Geometry: final body of the model. Coordinates: model frame, mm. Face numbers are marked on the shaded views. A direction names the side the tool comes from. Round coordinates to 2 decimals unless told otherwise and drop trailing zeros. Order: outer loops, then holes, each group sorted by start corner. A loop starts at its lowest first (then second) coordinate and runs counter-clockwise, first axis right, second up. Notation, with made-up numbers: M 18,-38.75 L 42,-38.75 A34 cw 42,-3.75 Z; hole C -34.75,89 d1. An arc over 180 degrees is marked long. Return JSON: item names as keys, results as strings. Group by question number.
Q1. Contact query for flat-ended pins moving along their axis: pin 1 (1.8 mm diameter, centred on x = -3.5, y = -0.5, fed in from -Z); pin 2 (4 mm diameter, centred on x = 1.5, z = -2.5, fed in from +Y); pin 3 (1.5 mm diameter, centred on x = 4, z = 1, fed in from -Y); pin 4 (4 mm diameter, centred on x = 4.5, y = 1.5, fed in from -Z). Output: stop coordinate, or through.
Q2. Access query for the marked faces 4, 5 and 6. Directions: +Z, -Z, +X, -X, +Y, -Y. A direction counts if a zero-diameter tool reaches every point of the face in a straight line with its end or side. Return the directions, or none.
Q3. Cut plane A-A on x = 9.25. Output: boundary loops of the cut face in (y, z), and give its area (3 significant figures).
Q4. Ray query, probe 1 along Z at (x, y) = (-3.5, 0); probe 2 along X at (y, z) = (-2.25, 1.25); probe 3 along X at (y, z) = (2, 0). Return the intervals inside material, ascending.
Q5. Mould query, pull axis Y, two halves, no side actions, for the marked faces 1, 2 and 3. Classes: released by +Y, released by -Y, zero draft, split by the parting line, or undercut.
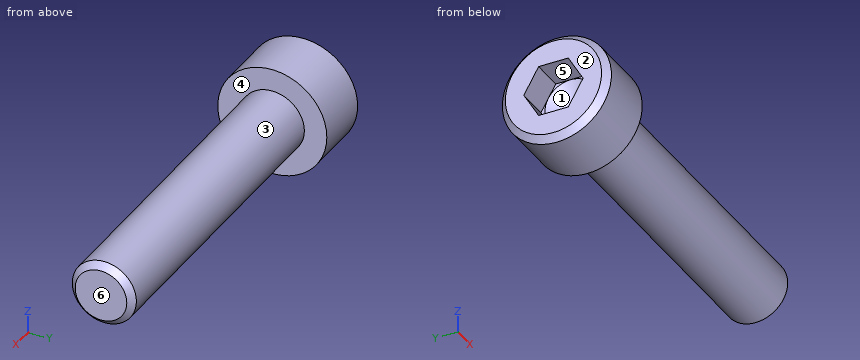
Autodesk Inventor part; units mm, degrees
ref_plane "bolt_XY" through (25, 0, 0) normal (1, 0, 0) x (0, 0, -1)
ref_plane "bolt_YZ" through (25, 0, 0) normal (0, 0, -1) x (0, 1, 0)
ref_plane "bolt_ZX" through (25, 0, 0) normal (0, 1, 0) x (1, 0, 0)
sketch "Sketch_1" plane through (0, 0, 0) normal (0, 0, 1) x (1, 0, 0)
  line L0 (25, 0) -> (-5, 0)
  line L1 (-5, 0) -> (-5, 3.75)
  line L2 (-5, 3.75) -> (-4.5, 4.25)
  line L3 (-4.5, 4.25) -> (0, 4.25)
  line L4 (0, 4.25) -> (0, 2.5)
  line L5 (0, 2.5) -> (24.5095, 2.5)
  line L6 (24.5095, 2.5) -> (25, 2.0095)
  line L7 (25, 2.0095) -> (25, 0)
  line L8 (25, 0) -> (-5, 0)
revolve "Revolution1" add sketch "Sketch_1" angle 360 about axis through (25, 0, 0) along (1, 0, 0)
thread "Thread1"
sketch "Sketch2" plane through (-5, 0, 0) normal (-1, 0, 0) x (0, 0, 1)
  point P0 (0, 0)
hole "Hole1" at (-5, 0, 0) direction (1, 0, 0) diameter 4 depth 2.5 tip angle 120
sketch "Sketch_3" plane through (-5, 0, 0) normal (1, 0, 0) x (0, 0, -1)
  line L0 (-2, -1.1547) -> (0, -2.3094)
  line L1 (0, -2.3094) -> (2, -1.1547)
  line L2 (2, -1.1547) -> (2, 1.1547)
  line L3 (2, 1.1547) -> (0, 2.3094)
  line L4 (0, 2.3094) -> (-2, 1.1547)
  line L5 (-2, 1.1547) -> (-2, -1.1547)
extrude "Extrusion1" cut sketch "Sketch_3" along normal blind 2.5
ref_plane "bolt_XY" through (25, 0, 0) normal (1, 0, 0) x (0, 0, -1)
ref_plane "bolt_YZ" through (25, 0, 0) normal (0, 0, -1) x (0, 1, 0)
ref_plane "bolt_ZX" through (25, 0, 0) normal (0, 1, 0) x (1, 0, 0)
ref_plane "nut_XY" through (0, 0, 0) normal (1, 0, 0) x (0, 0, -1)
ref_plane "nut_YZ" through (0, 0, 0) normal (0, 0, -1) x (0, 1, 0)
ref_plane "nut_ZX" through (0, 0, 0) normal (0, 1, 0) x (1, 0, 0)
properties part number "CBE5-25"
Result sheet:
{
 "1": {"pin 1": "stops at z = -4.25", "pin 2": "stops at y = 4.08", "pin 3": "stops at y = -2.49", "pin 4": "stops at z = -2.5"},
 "2": {"face 4": "+X", "face 5": "-X", "face 6": "+Z, -Z, +X, +Y, -Y"},
 "3": {"outline": "C 0,0 d5", "area": "19.6 mm²"},
 "4": {"probe 1": "z = -4.25 to -2, 2 to 4.25", "probe 2": "x = -5 to 0", "probe 3": "x = -2.5 to 25"},
 "5": {"face 1": "undercut", "face 2": "zero draft", "face 3": "split by the parting line"}
}
